Answer from the drawing. Dimensions are ordinates in mm from the lowest x, y and z of the part. A direction names the side the tool comes from. Round coordinates to 2 decimals unless told otherwise and drop trailing zeros. Order: outer loops, then holes, each group sorted by start corner. A loop starts at its lowest first (then second) coordinate and runs counter-clockwise, first axis right, second up. Notation, with made-up numbers: M 32,41.5 L 88,41.5 A15 cw 88,59.5 Z; hole C 10.25,84.5 d10. An arc over 180 degrees is marked long. Answer as a JSON object with one key per item and string values. Group by question number.
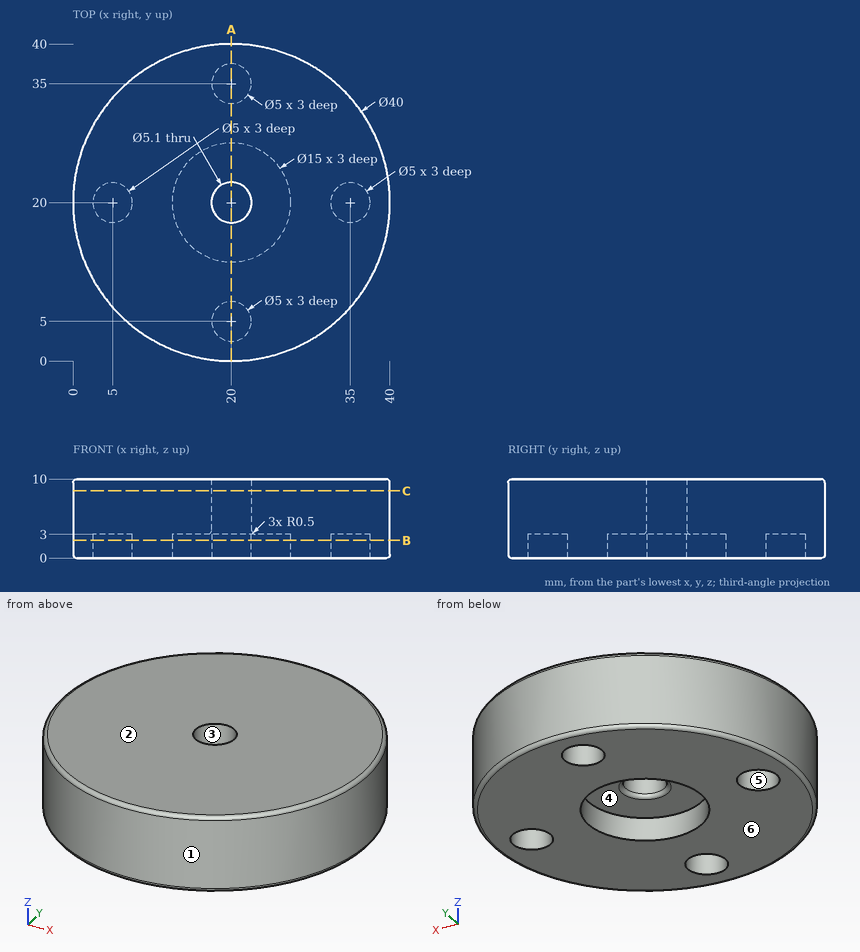
Item 1: The mould has two halves that part along Y. Classify the marked faces 1, 2, 3 and 4: +Y half, -Y half, draft (parallel to the pull), parting line (faces both ways), or undercut.
Item 2: Each of these flat-tipped pins is pushed along its axis until it touches: pin 1 (2 mm diameter, centred on y = 33.5, z = 1, fed in from +X); pin 2 (1.5 mm diameter, centred on x = 21, y = 4, fed in from -Z); pin 3 (1 mm diameter, centred on x = 25.5, z = 5.5, fed in from -Y). Where does it stop, or does it pass through?
Item 3: Find section B-B (z = 2.25). Give the vertices of the cut face in (x, y).
Item 4: Consider L1, parallel to Y at x = 20, z = 1.15; L2, parallel to Y at x = 20.5, z = 8; L3, parallel to Z at x = 34.5, y = 21. Determine where each line is inside the solid, lowest interval first.
Item 5: Find section C-C (z = 8.5). Give the vertices of the cut face in (x, y), and give its area (3 significant figures).
Item 6: Find section A-A (x = 20). Give the vertices of the cut face in (y, z), and give its area (3 significant figures).
Item 7: A tool of negligible diameter and unlimited length cuts with its end or side. For the marked faces 5 and 6, from which of +Z, -Z, +X, -X, +Y, -Y can it reach the whole face along a straight path? Write none if from no direction.
Responses:
{
 "1": {"face 1": "parting line", "face 2": "draft", "face 3": "undercut", "face 4": "undercut"},
 "2": {"pin 1": "stops at x = 35.61", "pin 2": "stops at z = 3", "pin 3": "stops at y = 0.64"},
 "3": {"outline": "C 20,20 d40; hole C 5,20 d5; hole C 20,20 d15; hole C 20,5 d5; hole C 20,35 d5; hole C 35,20 d5"},
 "4": {"L1": "y = 0 to 2.5, 7.5 to 12.5, 27.5 to 32.5, 37.5 to 40", "L2": "y = 0.01 to 17.5, 22.5 to 39.99", "L3": "z = 3 to 10"},
 "5": {"outline": "C 20,20 d40; hole C 20,20 d5.1", "area": "1,240 mm^2"},
 "6": {"outline": "M 0,0.5 A0.5 ccw 0.5,0 L 2.5,0 L 2.5,3 L 7.5,3 L 7.5,0 L 12.5,0 L 12.5,3 L 16.95,3 A0.5 ccw 17.45,3.5 L 17.45,10 L 0.5,10 A0.5 ccw 0,9.5 Z; M 22.55,3.5 A0.5 ccw 23.05,3 L 27.5,3 L 27.5,0 L 32.5,0 L 32.5,3 L 37.5,3 L 37.5,0 L 39.5,0 A0.5 ccw 40,0.5 L 40,9.5 A0.5 ccw 39.5,10 L 22.55,10 Z", "area": "289 mm^2"},
 "7": {"face 5": "-Z", "face 6": "-Z, +X, -X, +Y, -Y"}
}
